Source: CAD feature listing. Evaluate the final solid. Frame: model axes, mm. Face numbers are marked on the shaded views. A direction names the side the tool comes from. Round coordinates to 2 decimals unless told otherwise and drop trailing zeros. Order: outer loops, then holes, each group sorted by start corner. A loop starts at its lowest first (then second) coordinate and runs counter-clockwise, first axis right, second up. Notation, with made-up numbers: M 13.25,-13.75 L 36.25,-13.75 A6 cw 36.25,-4.75 Z; hole C 60.25,62.25 d4. An arc over 180 degrees is marked long. Use one line per item in the form item = value. Start each with the question number.
Q1. Pull-direction query (Z, two-part tool) for the marked faces 3, 4, 5 and 6; classes: pulls with the +Z half, pulls with the -Z half, needs draft (parallel to the pull), parting line crosses it, or undercut.
Q2. Contact query for flat-ended pins moving along their axis: pin 1 (10.5 mm diameter, centred on x = 140.5, z = -10.5, fed in from -Y); pin 2 (4 mm diameter, centred on x = 107.35, z = -28.65, fed in from -Y); pin 3 (1.6 mm diameter, centred on x = 22.5, z = -40.5, fed in from +Y). Output: stop coordinate, or through.
Q3. Reachability of the marked faces 1 and 2 from +Z, -Z, +X, -X, +Y, -Y: full face, straight path, thin tool, end or side. Return the list, or none.
Q4. Section C-C (z = -41). Return the cut outline in (x, y), plus the area to 3 significant figures.
Q5. Material intervals for probe 1 along X at (y, z) = (8.75, -10); probe 2 along X at (y, z) = (2.4, -70); probe 3 along X at (y, z) = (8.1, -51.35), sorted ascending.
Q6. Section B-B (y = 2). Give the number of separate pieces and of enclosed holes in the cut face, plus the area to 3 significant figures.
Q7. Section A-A (z = -70). Return the cut outline in (x, y), plus the area to 3 significant figures.
from build123d import *

# Parameters (mm, degrees)
SKETCH1_W            = 150
SKETCH1_H            = 80
BOSS_EXTRUDE1_DEPTH  = 10.5
SKETCH10_R           = 6.5
CUT_EXTRUDE8_DEPTH   = 5
WIREHOLES_REACH      = 172.324
SKETCH3_W            = 20
SKETCH3_H            = 10
SKETCH6_R            = 2.6
F_4AACUT_DEPTH       = 5.2
SKETCH7_R            = 2.6
F_2AACUT_DEPTH       = 5.2
SKETCH5_W            = 4.2
SKETCH5_H            = 20.2
ARDUINOMEGACUT_DEPTH = 5.2
SKETCH8_R            = 2.6
MPUCUT_DEPTH         = 5.2
CUT_EXTRUDE7_REACH   = 172.324
SKETCH9_R            = 2.6
SKETCH11_R           = 4
CUT_EXTRUDE9_DEPTH   = 0.5
SKETCH12_R           = 2.6
CUT_EXTRUDE10_DEPTH  = 5


with BuildPart() as part:
    # Sketch1 → Boss-Extrude1 (new body)
    with BuildSketch(Plane(origin=(0, 0, 0), x_dir=(1, 0, 0), z_dir=(0, 1, 0))):
        with Locations((75, 40)):
            Rectangle(SKETCH1_W, SKETCH1_H)
    extrude(amount=BOSS_EXTRUDE1_DEPTH)

    # Sketch10 → Cut-Extrude8 (cut)
    with BuildSketch(Plane(origin=(0, 10.5, 0), x_dir=(1, 0, 0), z_dir=(0, 1, 0))):
        with Locations(Location((10, 10, 0), (0, 0, 270))):
            Circle(SKETCH10_R)
        with Locations(Location((140, 10, 0), (0, 0, 270))):
            Circle(SKETCH10_R)
        with Locations(Location((10, 70, 0), (0, 0, 270))):
            Circle(SKETCH10_R)
        with Locations(Location((140, 70, 0), (0, 0, 270))):
            Circle(SKETCH10_R)
    cut_extrude8 = extrude(amount=-CUT_EXTRUDE8_DEPTH, mode=Mode.SUBTRACT)

    # Mirror1: Cut-Extrude8 across plane
    add(cut_extrude8.mirror(Plane.ZX.offset(5.25)), mode=Mode.SUBTRACT)

    # Sketch3 → WireHoles (cut, up to next)
    with BuildSketch(Plane(origin=(0, 10.5, 0), x_dir=(1, 0, 0), z_dir=(0, 1, 0)), mode=Mode.PRIVATE) as wireholes_sk1:
        with Locations((37.5, 10)):
            Rectangle(SKETCH3_W, SKETCH3_H)
    wireholes_tool1 = extrude(wireholes_sk1.sketch, amount=-WIREHOLES_REACH, mode=Mode.PRIVATE) & part.part
    # Sketch3 → WireHoles (cut, up to next)
    with BuildSketch(Plane(origin=(0, 10.5, 0), x_dir=(1, 0, 0), z_dir=(0, 1, 0)), mode=Mode.PRIVATE) as wireholes_sk2:
        with Locations((112.5, 10)):
            Rectangle(SKETCH3_W, SKETCH3_H)
    wireholes_tool2 = extrude(wireholes_sk2.sketch, amount=-WIREHOLES_REACH, mode=Mode.PRIVATE) & part.part
    add(wireholes_tool1.solids().sort_by_distance((37.5, 10.5, -10))[0], mode=Mode.SUBTRACT)
    add(wireholes_tool2.solids().sort_by_distance((112.5, 10.5, -10))[0], mode=Mode.SUBTRACT)

    # Sketch6 → 4AACut (cut)
    with BuildSketch(Plane(origin=(0, 10.5, 0), x_dir=(1, 0, 0), z_dir=(0, 1, 0))):
        with Locations(Location((21.4, 40, 0), (0, 0, 270))):
            Circle(SKETCH6_R)
        with Locations(Location((56.4, 40, 0), (0, 0, 90))):
            Circle(SKETCH6_R)
    extrude(amount=-F_4AACUT_DEPTH, mode=Mode.SUBTRACT)

    # Sketch7 → 2AACut (cut)
    with BuildSketch(Plane(origin=(0, 10.5, 0), x_dir=(1, 0, 0), z_dir=(0, 1, 0))):
        with Locations(Location((82.35, 51.35, 0), (0, 0, 270))):
            Circle(SKETCH7_R)
        with Locations(Location((107.35, 51.35, 0), (0, 0, 90))):
            Circle(SKETCH7_R)
        with Locations(Location((82.35, 28.65, 0), (0, 0, 90))):
            Circle(SKETCH7_R)
        with Locations(Location((107.35, 28.65, 0), (0, 0, 270))):
            Circle(SKETCH7_R)
    extrude(amount=-F_2AACUT_DEPTH, mode=Mode.SUBTRACT)

    # Sketch5 → ArduinoMegaCut (cut)
    with BuildSketch(Plane(origin=(0, 10.5, 0), x_dir=(1, 0, 0), z_dir=(0, 1, 0))):
        with Locations((50, 40)):
            Rectangle(SKETCH5_W, SKETCH5_H)
        with Locations((100, 40)):
            Rectangle(SKETCH5_W, SKETCH5_H)
    extrude(amount=-ARDUINOMEGACUT_DEPTH, mode=Mode.SUBTRACT)

    # Sketch8 → MPUCut (cut)
    with BuildSketch(Plane(origin=(0, 10.5, 0), x_dir=(1, 0, 0), z_dir=(0, 1, 0))):
        with Locations(Location((70, 4.8, 0), (0, 0, 270))):
            Circle(SKETCH8_R)
        with Locations(Location((80, 4.8, 0), (0, 0, 90))):
            Circle(SKETCH8_R)
    extrude(amount=-MPUCUT_DEPTH, mode=Mode.SUBTRACT)

    # Sketch9 → Cut-Extrude7 (cut, up to next)
    with BuildSketch(Plane(origin=(0, 10.5, 0), x_dir=(1, 0, 0), z_dir=(0, 1, 0)), mode=Mode.PRIVATE) as cut_extrude7_sk1:
        with Locations(Location((138.5, 45, 0), (0, 0, 270))):
            Circle(SKETCH9_R)
    cut_extrude7_tool1 = extrude(cut_extrude7_sk1.sketch, amount=-CUT_EXTRUDE7_REACH, mode=Mode.PRIVATE) & part.part
    # Sketch9 → Cut-Extrude7 (cut, up to next)
    with BuildSketch(Plane(origin=(0, 10.5, 0), x_dir=(1, 0, 0), z_dir=(0, 1, 0)), mode=Mode.PRIVATE) as cut_extrude7_sk2:
        with Locations(Location((138.5, 35, 0), (0, 0, 270))):
            Circle(SKETCH9_R)
    cut_extrude7_tool2 = extrude(cut_extrude7_sk2.sketch, amount=-CUT_EXTRUDE7_REACH, mode=Mode.PRIVATE) & part.part
    # Sketch9 → Cut-Extrude7 (cut, up to next)
    with BuildSketch(Plane(origin=(0, 10.5, 0), x_dir=(1, 0, 0), z_dir=(0, 1, 0)), mode=Mode.PRIVATE) as cut_extrude7_sk3:
        with Locations(Location((11.5, 45, 0), (0, 0, 270))):
            Circle(SKETCH9_R)
    cut_extrude7_tool3 = extrude(cut_extrude7_sk3.sketch, amount=-CUT_EXTRUDE7_REACH, mode=Mode.PRIVATE) & part.part
    # Sketch9 → Cut-Extrude7 (cut, up to next)
    with BuildSketch(Plane(origin=(0, 10.5, 0), x_dir=(1, 0, 0), z_dir=(0, 1, 0)), mode=Mode.PRIVATE) as cut_extrude7_sk4:
        with Locations(Location((11.5, 35, 0), (0, 0, 270))):
            Circle(SKETCH9_R)
    cut_extrude7_tool4 = extrude(cut_extrude7_sk4.sketch, amount=-CUT_EXTRUDE7_REACH, mode=Mode.PRIVATE) & part.part
    add(cut_extrude7_tool1.solids().sort_by_distance((138.5, 10.5, -45))[0], mode=Mode.SUBTRACT)
    add(cut_extrude7_tool2.solids().sort_by_distance((138.5, 10.5, -35))[0], mode=Mode.SUBTRACT)
    add(cut_extrude7_tool3.solids().sort_by_distance((11.5, 10.5, -45))[0], mode=Mode.SUBTRACT)
    add(cut_extrude7_tool4.solids().sort_by_distance((11.5, 10.5, -35))[0], mode=Mode.SUBTRACT)

    # Sketch11 → Cut-Extrude9 (cut)
    with BuildSketch(Plane(origin=(0, 5.5, 0), x_dir=(1, 0, 0), z_dir=(0, 1, 0))):
        with Locations(Location((10, 10, 0), (0, 0, 270))):
            Circle(SKETCH11_R)
        with Locations(Location((10, 70, 0), (0, 0, 90))):
            Circle(SKETCH11_R)
        with Locations(Location((140, 70, 0), (0, 0, 270))):
            Circle(SKETCH11_R)
        with Locations(Location((140, 10, 0), (0, 0, 90))):
            Circle(SKETCH11_R)
    extrude(amount=-CUT_EXTRUDE9_DEPTH, mode=Mode.SUBTRACT)

    # Sketch12 → Cut-Extrude10 (cut)
    with BuildSketch(Plane(origin=(0, 10.5, 0), x_dir=(1, 0, 0), z_dir=(0, 1, 0))):
        with Locations(Location((95, 75, 0), (0, 0, 270))):
            Circle(SKETCH12_R)
        with Locations(Location((105, 75, 0), (0, 0, 90))):
            Circle(SKETCH12_R)
    extrude(amount=-CUT_EXTRUDE10_DEPTH, mode=Mode.SUBTRACT)


solid = part.part
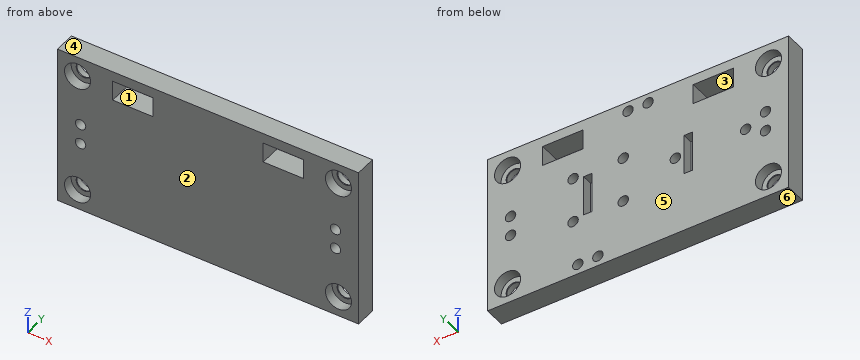
Results list:
q1.face_3 = undercut
q1.face_4 = pulls with the +Z half
q1.face_5 = needs draft
q1.face_6 = pulls with the -Z half
q2.pin_1 = 5
q2.pin_2 = 0
q2.pin_3 = 5.3
q3.face_1 = +Y, -Y
q3.face_2 = +Z, -Z, +X, -X, -Y
q4.outline = M 0,0 L 150,0 L 150,10.5 L 102.1,10.5 L 102.1,5.3 L 97.9,5.3 L 97.9,10.5 L 58.8,10.5 L 58.8,5.3 L 54,5.3 L 54,10.5 L 52.1,10.5 L 52.1,5.3 L 47.9,5.3 L 47.9,10.5 L 23.8,10.5 L 23.8,5.3 L 19,5.3 L 19,10.5 L 0,10.5 Z
q4.area = 1,480 mm2
q5.probe_1 = 0 to 3.5, 16.5 to 27.5, 47.5 to 102.5, 122.5 to 133.5, 146.5 to 150
q5.probe_2 = 0 to 3.5, 16.5 to 133.5, 146.5 to 150
q5.probe_3 = 0 to 79.75, 84.95 to 104.75, 109.95 to 150
q6.separate_pieces = 1
q6.enclosed_holes = 10
q6.area = 11,000 mm2
q7.outline = M 0,0 L 3.5,0 L 3.5,5 L 6,5 L 6,5.5 L 3.5,5.5 L 3.5,10.5 L 0,10.5 Z; M 14,5 L 16.5,5 L 16.5,0 L 133.5,0 L 133.5,5 L 136,5 L 136,5.5 L 133.5,5.5 L 133.5,10.5 L 16.5,10.5 L 16.5,5.5 L 14,5.5 Z; M 144,5 L 146.5,5 L 146.5,0 L 150,0 L 150,10.5 L 146.5,10.5 L 146.5,5.5 L 144,5.5 Z
q7.area = 1,310 mm2
